Check sheet for the modelled part. Datum: model origin and axes. Units: mm. Coordinates: 2 decimals unless noted, no trailing zeros. Loops run counter-clockwise (first coordinate to the right, second up) from the corner with the lowest first, then second, coordinate; pieces in that order, holes last. Notation, with made-up numbers: M -11,-21 L 37,-21 A26 cw 37,9 Z; hole C 26,48.25 d1. An arc over 180 degrees is marked long. Write each question's results on one line, items separated by ' | '. Start each with the question number.
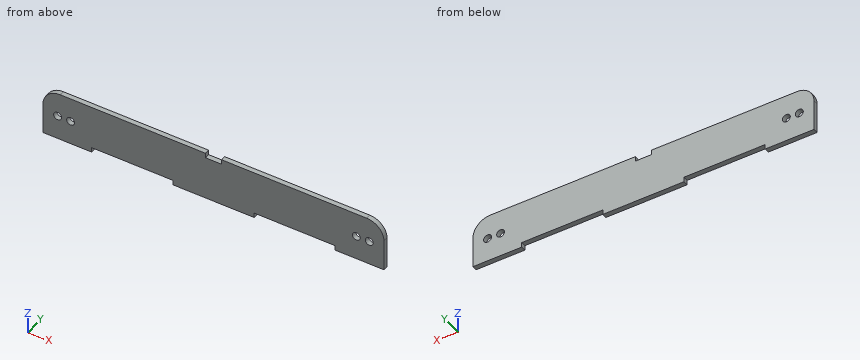
from build123d import *

# Parameters (mm, degrees)
SKETCH1_W               = 210
SKETCH1_H               = 30
BOSS_EXTRUDE1_DEPTH     = 3
CUT_EXTRUDE1_DEPTH      = 107.108435103
CUT_EXTRUDE1_DEPTH_BACK = 107.108435103
SKETCH2_W               = 50
SKETCH2_H               = 3
CUT_EXTRUDE2_DEPTH      = 107.108435103
CUT_EXTRUDE2_DEPTH_BACK = 107.108435103
CUT_EXTRUDE4_DEPTH      = 107.108435103
CUT_EXTRUDE4_DEPTH_BACK = 107.108435103
SKETCH5_R               = 2.45
CUT_EXTRUDE5_DEPTH      = 107.108435103
CUT_EXTRUDE5_DEPTH_BACK = 107.108435103


with BuildPart() as part:
    # Sketch1 → Boss-Extrude1 (new body)
    with BuildSketch(Plane(origin=(0, 0, 0), x_dir=(1, 0, 0), z_dir=(0, 1, 0))):
        Rectangle(SKETCH1_W, SKETCH1_H)
    extrude(amount=BOSS_EXTRUDE1_DEPTH)

    # Sketch2 → Cut-Extrude1 (cut, two sides: drawn at the far end of the back side and taken through both)
    with BuildSketch(Plane(origin=(0, 3, 0), x_dir=(1, 0, 0), z_dir=(0, 1, 0)).offset(-CUT_EXTRUDE1_DEPTH_BACK)):
        with Locations((-50, 13.5)):
            Rectangle(SKETCH2_W, SKETCH2_H)
        with Locations((50, 13.5)):
            Rectangle(SKETCH2_W, SKETCH2_H)
    extrude(amount=CUT_EXTRUDE1_DEPTH + CUT_EXTRUDE1_DEPTH_BACK, mode=Mode.SUBTRACT)

    # Sketch3 → Cut-Extrude2 (cut, two sides: drawn at the far end of the back side and taken through both)
    with BuildSketch(Plane.XZ.offset(-CUT_EXTRUDE2_DEPTH_BACK)):
        Polygon((0, 15), (5, 15), (5, 12), (-5, 12), (-5, 15), align=None)
    extrude(amount=CUT_EXTRUDE2_DEPTH + CUT_EXTRUDE2_DEPTH_BACK, mode=Mode.SUBTRACT)

    # Sketch5 → Cut-Extrude4 (cut, two sides: drawn at the far end of the back side and taken through both)
    with BuildSketch(Plane(origin=(0, 0, 0), x_dir=(1, 0, 0), z_dir=(0, 1, 0)).offset(-CUT_EXTRUDE4_DEPTH_BACK)):
        with Locations(Location((-96, 0, 0), (0, 0, 270))):
            Circle(SKETCH5_R)
        with Locations(Location((-88, 0, 0), (0, 0, 270))):
            Circle(SKETCH5_R)
        with Locations(Location((88, 0, 0), (0, 0, 270))):
            Circle(SKETCH5_R)
        with Locations(Location((96, 0, 0), (0, 0, 270))):
            Circle(SKETCH5_R)
    extrude(amount=CUT_EXTRUDE4_DEPTH + CUT_EXTRUDE4_DEPTH_BACK, mode=Mode.SUBTRACT)

    # Sketch6 → Cut-Extrude5 (cut, two sides: drawn at the far end of the back side and taken through both)
    with BuildSketch(Plane(origin=(0, 0, 0), x_dir=(1, 0, 0), z_dir=(0, 1, 0)).offset(-CUT_EXTRUDE5_DEPTH_BACK)):
        with BuildLine():
            Line((-105, -4.393398282), (-105, -15))
            Line((-105, -15), (-94.393398282, -15))
            ThreePointArc((-94.393398282, -15), (-101.893398282, -11.893398282), (-105, -4.393398282))
        make_face()
        with BuildLine():
            Line((105, -15), (94.393398282, -15))
            ThreePointArc((94.393398282, -15), (101.893398282, -11.893398282), (105, -4.393398282))
            Line((105, -4.393398282), (105, -15))
        make_face()
    extrude(amount=CUT_EXTRUDE5_DEPTH + CUT_EXTRUDE5_DEPTH_BACK, mode=Mode.SUBTRACT)


solid = part.part
Item 1: Depth check by flat-ended pin: P1, Ø1.5, axis at y = 1.5, z = 13, coming from the -X side. Enter the tip coordinate at first touch or a pass-through.
Item 2: Section check B-B (z = 0). Record the cut outline in (x, y), plus the area to 3 significant figures.
Item 3: Section check C-C (x = -88). Record the cut outline in (y, z), plus the area to 3 significant figures.
Item 4: Thickness scan on line 1 (X direction, y = 1.7, z = 0); line 2 (Z direction, x = 88, y = 1.95); line 3 (X direction, y = 0.5, z = -1.25). Record the ranges inside material, lowest first.
Item 5: Section check A-A (y = 1.9). Record the cut outline in (x, z), plus the area to 3 significant figures.
Computed values:
1) P1: stops at x = -101.52
2) outline: M -105,0 L -98.45,0 L -98.45,3 L -105,3 Z; M -93.55,0 L -90.45,0 L -90.45,3 L -93.55,3 Z; M -85.55,0 L 85.55,0 L 85.55,3 L -85.55,3 Z; M 90.45,0 L 93.55,0 L 93.55,3 L 90.45,3 Z; M 98.45,0 L 105,0 L 105,3 L 98.45,3 Z | area: 571 mm²
3) outline: M 0,-15 L 3,-15 L 3,-2.45 L 0,-2.45 Z; M 0,2.45 L 3,2.45 L 3,15 L 0,15 Z | area: 75.3 mm²
4) line 1: x = -105 to -98.45, -93.55 to -90.45, -85.55 to 85.55, 90.45 to 93.55, 98.45 to 105 | line 2: z = -15 to -2.45, 2.45 to 15 | line 3: x = -105 to -98.11, -93.89 to -90.11, -85.89 to 85.89, 90.11 to 93.89, 98.11 to 105
5) outline: M -105,-15 L -75,-15 L -75,-12 L -25,-12 L -25,-15 L 25,-15 L 25,-12 L 75,-12 L 75,-15 L 105,-15 L 105,4.39 A10.61 ccw 94.39,15 L 5,15 L 5,12 L -5,12 L -5,15 L -94.39,15 A10.61 ccw -105,4.39 Z; hole C -96,0 d4.9; hole C -88,0 d4.9; hole C 88,0 d4.9; hole C 96,0 d4.9 | area: 5,850 mm²
